Part print with two shaded views. Sizes in mm from the minimum x, y, z corner. Round coordinates to 2 decimals unless told otherwise and drop trailing zeros. Loops run counter-clockwise (first coordinate to the right, second up) from the corner with the lowest first, then second, coordinate; pieces in that order, holes last. Notation, with made-up numbers: (-9, 15) - (6, 15) arc R23 cw to (6, 51) - close; hole circle Ø1 at (64, 9). An arc over 180 degrees is marked (long way). Write each question's results on one line, items separated by ' | '. Start each with the question number.
(1) Cut at D-D, the plane x = 48. List the corners of the cut face in (y, z).
(2) Mould opens along Y. For the marked faces 1, 2 and 3 say: released by +Y, released by -Y, zero draft, split by the parting line, or undercut.
(3) Cut at B-B, the plane x = 19.5. List the corners of the cut face in (y, z).
(4) Cut at C-C, the plane y = 7. List the corners of the cut face in (x, z).
(5) Flat gauge pins, fed straight in: P1, Ø1.5, axis at x = 45, y = 22, coming from the +Z side; P2, Ø5, axis at y = 13.5, z = 10.5, coming from the +X side (3 decimals); P3, Ø2, axis at y = 12.5, z = 10, coming from the -X side (3 decimals); P4, Ø7.5, axis at x = 15.875, y = 12.7, coming from the -Z side. Where does each tip first touch, or does it go through?
(6) Drill centre lines: L1, parallel to Z at x = 8, y = 2.5; L2, parallel to X at y = 18.25, z = 3; L3, parallel to X at y = 12.5, z = 9. Where is each one in solid material? Low to high.
(7) Cut at A-A, the plane z = 4.25. List the corners of the cut face in (x, y) (3 decimals).
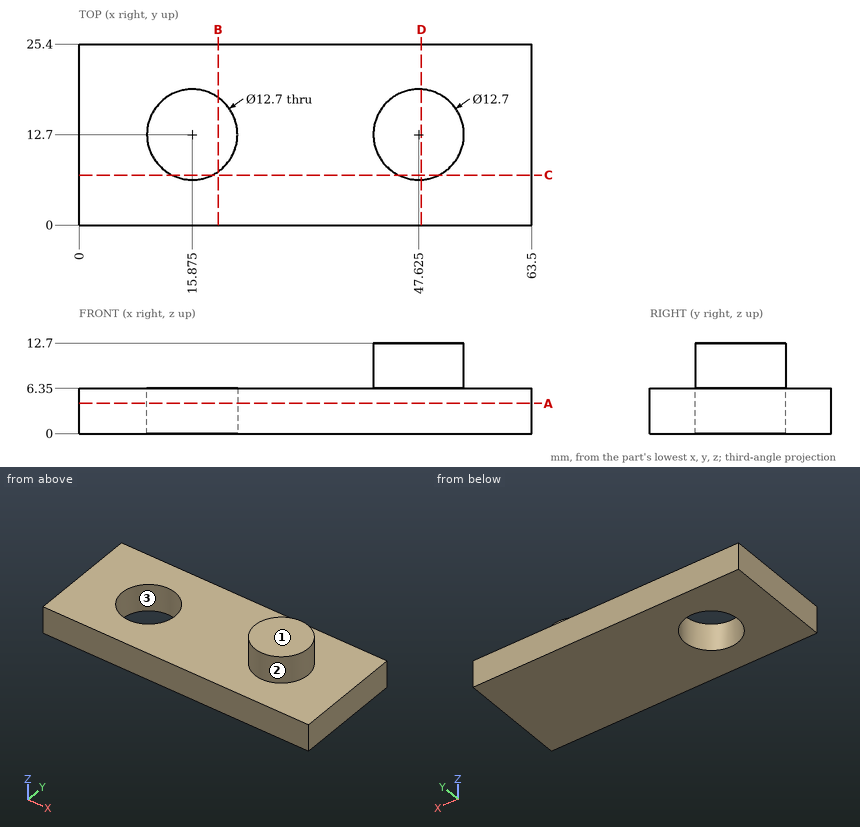
A:
1) outline: (0, 0) - (25.4, 0) - (25.4, 6.35) - (19.04, 6.35) - (19.04, 12.7) - (6.36, 12.7) - (6.36, 6.35) - (0, 6.35) - close
2) face 1: zero draft | face 2: split by the parting line | face 3: undercut
3) outline: (0, 0) - (7.49, 0) - (7.49, 6.35) - (0, 6.35) - close; (17.91, 0) - (25.4, 0) - (25.4, 6.35) - (17.91, 6.35) - close
4) outline: (0, 0) - (13.08, 0) - (13.08, 6.35) - (0, 6.35) - close; (18.67, 0) - (63.5, 0) - (63.5, 6.35) - (50.42, 6.35) - (50.42, 12.7) - (44.83, 12.7) - (44.83, 6.35) - (18.67, 6.35) - close
5) P1: z = 6.35 | P2: x = 53.975 | P3: x = 41.275 | P4: through
6) L1: 0 to 6.35 | L2: 0 to 12.79, 18.96 to 63.5 | L3: 41.28 to 53.97
7) outline: (0, 0) - (63.5, 0) - (63.5, 25.4) - (0, 25.4) - close; hole circle Ø12.7 at (15.875, 12.7)
